```python
from build123d import *

# Parameters (mm, degrees)
F0_W      = 152.4
F0_H      = 152.4
F1_DEPTH  = 152.4
F2_R      = 5.08
F3_R      = 38.6645331573
F4_DEPTH  = 102.362
F5_R      = 15.7820289437
F6_DEPTH  = 56.134
F7_R      = 5.08
F9_D      = 15.24
F10_DEPTH = 25.4


with BuildPart() as f1:
    # F0 (on Top) → F1 (new body)
    with BuildSketch(Plane.XY):
        Rectangle(F0_W, F0_H)
    extrude(amount=F1_DEPTH)

    # F2
    f2_edges = [f1.edges().sort_by_distance(p)[0] for p in [
        (76.2, 0, 152.4),
        (0, 76.2, 152.4),
        (-76.2, 0, 152.4),
        (0, -76.2, 152.4),
    ]]
    fillet(f2_edges, radius=F2_R)

    # F3 (on face) → F4 (join)
    with BuildSketch(Plane.XZ.offset(76.2)):
        with Locations((0, 69.6934089065)):
            Circle(F3_R)
    extrude(amount=F4_DEPTH)

    # F5 (on face) → F6 (join)
    with BuildSketch(Plane.XZ.offset(178.562)):
        with Locations((0, 69.6934089065)):
            Circle(F5_R)
    extrude(amount=F6_DEPTH)

    # F7
    f7_edges = [f1.edges().sort_by_distance(p)[0] for p in [
        (-15.782029, -234.696, 69.693409),
        (-15.782029, -178.562, 69.693409),
        (-38.664533, -178.562, 69.693409),
        (-38.664533, -76.2, 69.693409),
    ]]
    fillet(f7_edges, radius=F7_R)

    # F9 (through all)
    with Locations(Plane.XZ.offset(234.696)):
        with Locations((0, 69.6934089065)):
            Hole(F9_D / 2)

    # F10 (add): a face of the model
    f10_faces = [f1.faces().sort_by_distance(p)[0] for p in [
        (-10.3993298541, -234.696, 69.6934089065),
    ]]
    extrude(f10_faces, amount=F10_DEPTH)


solid = f1.part
```
Here's how the part is built. I have some questions about the finished solid (model axes, mm). A direction names the side the tool comes from. Give positions to 0.01 mm unless a question says otherwise; leave off trailing zeros. Write each loop counter-clockwise with the first axis right and the second up, starting at its lowest first coordinate (ties: lowest second). Pieces come first, ordered by that corner, then holes. Notation, with made-up numbers: M 33,-7.5 L 82,-7.5 A10 ccw 82,10.5 Z; hole C 10,17 d10. An arc over 180 degrees is marked long. Put each result on its own line as item: value. Start each with the question number.
Item 1: I need wall thicknesses on L1, parallel to Z at x = 0, y = -48; L2, parallel to Z at x = 0, y = -149; L3, parallel to Y at x = 55, z = 22. Which ranges of each line are inside material? Lowest first, please. Write a range as from..to.
Item 2: Will these pins go through, and if not, where does the flat tip stop? pin 1 (4 mm diameter, centred on x = -7, y = -173, fed in from -Z); pin 2 (5 mm diameter, centred on x = -15, z = 130, fed in from -Y).
Item 3: If we section it at B-B, the plane z = 120.5: Write out the boundary of the cut face in (x, y).
Item 4: If we section it at C-C, the plane x = 57: Write out the boundary of the cut face in (y, z).
Item 5: If we section it at A-A, the plane x = 0: Write out the boundary of the cut face in (y, z).
Item 6: On a 3-axis mill with a long thin cutter (end or side, diameter ignored), from which of +Z, -Z, +X, -X, +Y, -Y can I reach the whole of each face in a straight line? I mean faces 1 (the flat face through (-15.4, -178.562, 55.2)), 2 (the flat face through (-76.2, -1, 73)). Say none if no direction works.
Item 7: Thinking about a two-plate mould opening in Z: for faces 3 (the flat face through (33, -76.2, 105)), 4 (the cylindrical face through (1.652, -89.594, 62.255)), 5 (the cylindrical face through (-5.03, -126.74, 108.03)), which applies, +Z half, -Z half, draft (parallel to the pull), parting line (faces both ways), or undercut?
Item 8: If we section it at D-D, the plane y = -215: Write out the boundary of the cut face in (x, z), then the cut area to 3 significant figures.
Values:
1. L1: 0..62.07, 77.31..152.4
1. L2: 31.03..62.07, 77.31..108.36
1. L3: -76.2..76.2
2. pin 1: z = 31.35
2. pin 2: y = -76.2
3. outline: M -76.2,-76.2 L 76.2,-76.2 L 76.2,76.2 L -76.2,76.2 Z
4. outline: M -76.2,0 L 76.2,0 L 76.2,147.32 A5.08 ccw 71.12,152.4 L -71.12,152.4 A5.08 ccw -76.2,147.32 Z
5. outline: M -260.1,58.99 L -234.7,58.99 A5.08 ccw -229.62,53.91 L -183.64,53.91 A5.08 cw -178.56,48.83 L -178.56,36.11 A5.08 ccw -173.48,31.03 L -81.28,31.03 A5.08 cw -76.2,25.95 L -76.2,0 L 76.2,0 L 76.2,62.07 L -260.1,62.07 Z; M -260.1,77.31 L 76.2,77.31 L 76.2,147.32 A5.08 ccw 71.12,152.4 L -71.12,152.4 A5.08 ccw -76.2,147.32 L -76.2,113.44 A5.08 cw -81.28,108.36 L -173.48,108.36 A5.08 ccw -178.56,103.28 L -178.56,90.56 A5.08 cw -183.64,85.48 L -229.62,85.48 A5.08 ccw -234.7,80.4 L -260.1,80.4 Z
6. face 1: -Y
6. face 2: +Z, -Z, -X, +Y, -Y
7. face 3: draft
7. face 4: undercut
7. face 5: parting line
8. outline: C 0,69.69 d31.56; hole C 0,69.69 d15.24
8. area: 600 mm²
